```python
from build123d import *

# Parameters (mm, degrees)
SKETCH_1_W               = 27.5
SKETCH_1_H               = 22.5
EXTRUDE_1_DEPTH          = 17.8
CUT_EXTRUDE_1_DEPTH      = 26.148856833
CUT_EXTRUDE_1_DEPTH_BACK = 26.148856833
SKETCH_3_W               = 15.5
SKETCH_3_H               = 12.2
CUT_EXTRUDE_2_DEPTH      = 26.148856833
EXTRUDE_2_DEPTH          = 5.1
EXTRUDE_2_DEPTH_BACK     = 5.1
EXTRUDE_3_DEPTH          = 0.99
EXTRUDE_4_DEPTH          = 0.99
EXTRUDE_5_DEPTH          = 3.01
SKETCH_8_R               = 0.4
EXTRUDE_6_DEPTH          = 2
SKETCH_9_W               = 27.7
SKETCH_9_H               = 18
SKETCH_9_W_2             = 27.5
SKETCH_9_H_2             = 17.8
EXTRUDE_7_DEPTH          = 8.5


with BuildPart() as part:
    # Эскиз1 → Бобышка-Вытянуть1 (new body)
    with BuildSketch(Plane(origin=(0, 0, 0), x_dir=(1, 0, 0), z_dir=(0, 1, 0))):
        Rectangle(SKETCH_1_W, SKETCH_1_H)
    extrude(amount=EXTRUDE_1_DEPTH)

    # Эскиз3 → Вырез-Вытянуть1 (cut, two sides: drawn at the far end of the back side and taken through both)
    with BuildSketch(Plane.XY.offset(-CUT_EXTRUDE_1_DEPTH_BACK)):
        with Locations((0, 8.9)):
            Rectangle(SKETCH_3_W, SKETCH_3_H)
    extrude(amount=CUT_EXTRUDE_1_DEPTH + CUT_EXTRUDE_1_DEPTH_BACK, mode=Mode.SUBTRACT)

    # Эскиз4 → Вырез-Вытянуть2 (cut, through all)
    with BuildSketch(Plane(origin=(0, 0, 0), x_dir=(1, 0, 0), z_dir=(0, 1, 0))):
        Polygon((-4.5, 11.25), (-2.75, 8.75), (2.75, 8.75), (4.5, 11.25), align=None)
        Polygon((4.5, -11.25), (-4.5, -11.25), (-2.75, -8.75), (2.75, -8.75), align=None)
    extrude(amount=CUT_EXTRUDE_2_DEPTH, mode=Mode.SUBTRACT)

    # Эскиз2 → Бобышка-Вытянуть2 (add, two sides: drawn at the far end of the back side and taken through both)
    with BuildSketch(Plane(origin=(0, 8.9, 0), x_dir=(1, 0, 0), z_dir=(0, 1, 0)).offset(-EXTRUDE_2_DEPTH_BACK)):
        with BuildLine():
            Line((-10, -2.5), (-10, 2.5))
            ThreePointArc((-10, 2.5), (0, 12.5), (10, 2.5))
            Line((10, 2.5), (10, -2.5))
            ThreePointArc((10, -2.5), (0, -12.5), (-10, -2.5))
        make_face()
    extrude(amount=EXTRUDE_2_DEPTH + EXTRUDE_2_DEPTH_BACK)

    # Эскиз5 → Бобышка-Вытянуть3 (add)
    with BuildSketch(Plane.XZ.offset(-3.8)):
        with BuildLine():
            Line((7, 11.75), (7, -11.75))
            ThreePointArc((7, -11.75), (6.853553391, -12.103553391), (6.5, -12.25))
            Line((6.5, -12.25), (2.75, -12.25))
            Line((2.75, -12.25), (2.084693312, -9.145235456))
            ThreePointArc((2.084693312, -9.145235456), (1.910130877, -8.861166956), (1.595792105, -8.75))
            Line((1.595792105, -8.75), (-1.595792105, -8.75))
            ThreePointArc((-1.595792105, -8.75), (-1.910130877, -8.861166956), (-2.084693312, -9.145235456))
            Line((-2.084693312, -9.145235456), (-2.75, -12.25))
            Line((-2.75, -12.25), (-6.5, -12.25))
            ThreePointArc((-6.5, -12.25), (-6.853553391, -12.103553391), (-7, -11.75))
            Line((-7, -11.75), (-7, 11.75))
            ThreePointArc((-7, 11.75), (-6.853553391, 12.103553391), (-6.5, 12.25))
            Line((-6.5, 12.25), (-2.75, 12.25))
            Line((-2.75, 12.25), (-2.084693312, 9.145235456))
            ThreePointArc((-2.084693312, 9.145235456), (-1.910130877, 8.861166956), (-1.595792105, 8.75))
            Line((-1.595792105, 8.75), (1.595792105, 8.75))
            ThreePointArc((1.595792105, 8.75), (1.910130877, 8.861166956), (2.084693312, 9.145235456))
            Line((2.084693312, 9.145235456), (2.75, 12.25))
            Line((2.75, 12.25), (6.5, 12.25))
            ThreePointArc((6.5, 12.25), (6.853553391, 12.103553391), (7, 11.75))
        make_face()
    extrude(amount=EXTRUDE_3_DEPTH)

    # Эскиз6 → Бобышка-Вытянуть4 (add)
    with BuildSketch(Plane(origin=(0, 14, 0), x_dir=(1, 0, 0), z_dir=(0, 1, 0))):
        with BuildLine():
            Line((-7, -12.75), (-7, 12.75))
            ThreePointArc((-7, 12.75), (-6.853553391, 13.103553391), (-6.5, 13.25))
            Line((-6.5, 13.25), (-6.2, 13.25))
            ThreePointArc((-6.2, 13.25), (-5.7, 12.75), (-5.2, 13.25))
            Line((-5.2, 13.25), (-3.25, 13.25))
            ThreePointArc((-3.25, 13.25), (-2.896446609, 13.103553391), (-2.75, 12.75))
            Line((-2.75, 12.75), (-2.75, 8.75))
            Line((-2.75, 8.75), (2.75, 8.75))
            Line((2.75, 8.75), (2.75, 12.75))
            ThreePointArc((2.75, 12.75), (2.896446609, 13.103553391), (3.25, 13.25))
            Line((3.25, 13.25), (5.2, 13.25))
            ThreePointArc((5.2, 13.25), (5.7, 12.75), (6.2, 13.25))
            Line((6.2, 13.25), (6.5, 13.25))
            ThreePointArc((6.5, 13.25), (6.853553391, 13.103553391), (7, 12.75))
            Line((7, 12.75), (7, -12.75))
            ThreePointArc((7, -12.75), (6.853553391, -13.103553391), (6.5, -13.25))
            Line((6.5, -13.25), (6.2, -13.25))
            ThreePointArc((6.2, -13.25), (5.7, -12.75), (5.2, -13.25))
            Line((5.2, -13.25), (3.25, -13.25))
            ThreePointArc((3.25, -13.25), (2.896446609, -13.103553391), (2.75, -12.75))
            Line((2.75, -12.75), (2.75, -8.75))
            Line((2.75, -8.75), (-2.75, -8.75))
            Line((-2.75, -8.75), (-2.75, -12.75))
            ThreePointArc((-2.75, -12.75), (-2.896446609, -13.103553391), (-3.25, -13.25))
            Line((-3.25, -13.25), (-5.2, -13.25))
            ThreePointArc((-5.2, -13.25), (-5.7, -12.75), (-6.2, -13.25))
            Line((-6.2, -13.25), (-6.5, -13.25))
            ThreePointArc((-6.5, -13.25), (-6.853553391, -13.103553391), (-7, -12.75))
        make_face()
    extrude(amount=EXTRUDE_4_DEPTH)

    # Эскиз7 → Бобышка-Вытянуть5 (add)
    with BuildSketch(Plane(origin=(0, 14.99, 0), x_dir=(1, 0, 0), z_dir=(0, 1, 0))):
        with BuildLine():
            Line((-7, 11.25), (-2.75, 11.25))
            Line((-2.75, 11.25), (-2.75, 12.75))
            ThreePointArc((-2.75, 12.75), (-2.896446609, 13.103553391), (-3.25, 13.25))
            Line((-3.25, 13.25), (-5.2, 13.25))
            ThreePointArc((-5.2, 13.25), (-5.7, 12.75), (-6.2, 13.25))
            Line((-6.2, 13.25), (-6.5, 13.25))
            ThreePointArc((-6.5, 13.25), (-6.853553391, 13.103553391), (-7, 12.75))
            Line((-7, 12.75), (-7, 11.25))
        make_face()
        with BuildLine():
            Line((7, 11.25), (2.75, 11.25))
            Line((2.75, 11.25), (2.75, 12.75))
            ThreePointArc((2.75, 12.75), (2.896446609, 13.103553391), (3.25, 13.25))
            Line((3.25, 13.25), (5.2, 13.25))
            ThreePointArc((5.2, 13.25), (5.7, 12.75), (6.2, 13.25))
            Line((6.2, 13.25), (6.5, 13.25))
            ThreePointArc((6.5, 13.25), (6.853553391, 13.103553391), (7, 12.75))
            Line((7, 12.75), (7, 11.25))
        make_face()
        with BuildLine():
            Line((7, -11.25), (2.75, -11.25))
            Line((2.75, -11.25), (2.75, -12.75))
            ThreePointArc((2.75, -12.75), (2.896446609, -13.103553391), (3.25, -13.25))
            Line((3.25, -13.25), (5.2, -13.25))
            ThreePointArc((5.2, -13.25), (5.7, -12.75), (6.2, -13.25))
            Line((6.2, -13.25), (6.5, -13.25))
            ThreePointArc((6.5, -13.25), (6.853553391, -13.103553391), (7, -12.75))
            Line((7, -12.75), (7, -11.25))
        make_face()
        with BuildLine():
            Line((-7, -11.25), (-2.75, -11.25))
            Line((-2.75, -11.25), (-2.75, -12.75))
            ThreePointArc((-2.75, -12.75), (-2.896446609, -13.103553391), (-3.25, -13.25))
            Line((-3.25, -13.25), (-5.2, -13.25))
            ThreePointArc((-5.2, -13.25), (-5.7, -12.75), (-6.2, -13.25))
            Line((-6.2, -13.25), (-6.5, -13.25))
            ThreePointArc((-6.5, -13.25), (-6.853553391, -13.103553391), (-7, -12.75))
            Line((-7, -12.75), (-7, -11.25))
        make_face()
    extrude(amount=EXTRUDE_5_DEPTH)

    # Эскиз8 → Бобышка-Вытянуть6 (add)
    with BuildSketch(Plane(origin=(0, 18, 0), x_dir=(1, 0, 0), z_dir=(0, 1, 0))):
        with Locations(Location((4, -12.25, 0), (0, 0, 90))):
            Circle(SKETCH_8_R)
        with Locations(Location((-4, -12.25, 0), (0, 0, 90))):
            Circle(SKETCH_8_R)
        with Locations(Location((-4, 12.25, 0), (0, 0, 90))):
            Circle(SKETCH_8_R)
        with Locations(Location((4, 12.25, 0), (0, 0, 90))):
            Circle(SKETCH_8_R)
    extrude(amount=EXTRUDE_6_DEPTH)

    # Эскиз9 → Бобышка-Вытянуть7 (add, symmetric)
    with BuildSketch(Plane.XY):
        with Locations((0, 8.9)):
            Rectangle(SKETCH_9_W, SKETCH_9_H)
        with Locations((0, 8.9)):
            Rectangle(SKETCH_9_W_2, SKETCH_9_H_2, mode=Mode.SUBTRACT)
    extrude(amount=EXTRUDE_7_DEPTH, both=True)


solid = part.part
```
Geometry: final body of the model. Coordinates: model frame, mm. A direction names the side the tool comes from. Give positions to 0.01 mm unless a question says otherwise; leave off trailing zeros. Write each loop counter-clockwise with the first axis right and the second up, starting at its lowest first coordinate (ties: lowest second). Pieces come first, ordered by that corner, then holes.
1. Pin query (flat end, axial travel): P1, Ø1.4, axis at x = 0, y = 15.5, coming from the -Z side; P2, Ø12, axis at x = -7, z = -4.5, coming from the +Y side; P3, Ø4, axis at x = 4, z = -11.5, coming from the -Y side. Return the tip coordinate at first contact, or that it passes through.
2. Reachability of faces 5 (the flat face through (2.422, 3.312, -10.719)), 6 (the flat face through (-3.64, 1.38, 10.02)), 7 (the flat face through (-5, 3, 12.25)) from +Z, -Z, +X, -X, +Y, -Y: full face, straight path, thin tool, end or side. Return the list, or none.
3. Section query C-C, the plane y = 6.5. Return loops of the section in (x, z).
4. Line query: probe 1 along Z at (x, y) = (3.75, 17.25); probe 2 along Z at (x, y) = (4, 19.25); probe 3 along X at (y, z) = (15.25, 12.25). Output: solid intervals per line, ascending.
5. Section query B-B, the plane z = 6. Return loops of the section in (x, y).
6. Section query A-A, the plane x = -0.25. Return loops of the section in (y, z).
7. Section query D-D, the plane x = -5.7. Count the separate pieces of the cut face and the enclosed holes in it, then the cut area to 3 significant figures.
8. Draft query along X for faces 1 (the flat face through (5, 14, -12)), 2 (the flat face through (10, 9, 11.25)), 3 (the flat face through (-13.85, 9, 0)), 4 (the cylindrical face through (3.88, 18.99, 11.87)). Return one class per face: released by +X, released by -X, zero draft, split by the parting line, or undercut.
Computed:
1. P1: stops at z = -8.75
1. P2: stops at y = 17.9
1. P3: stops at y = 0
2. face 5: -Z, -Y
2. face 6: +Z, -Y
2. face 7: +Z, +X, -X, -Y
3. outline: (-13.85, -8.5) - (-13.75, -8.5) - (-13.75, -11.25) - (-7.75, -11.25) - (-7.75, -8.82) arc R10 ccw to (7.75, -8.82) - (7.75, -11.25) - (13.75, -11.25) - (13.75, -8.5) - (13.85, -8.5) - (13.85, 8.5) - (13.75, 8.5) - (13.75, 11.25) - (7.75, 11.25) - (7.75, 8.82) arc R10 ccw to (-7.75, 8.82) - (-7.75, 11.25) - (-13.75, 11.25) - (-13.75, 8.5) - (-13.85, 8.5) - close
4. probe 1: z = -13.25 to -11.25, -10.18 to 10.18, 11.25 to 13.25
4. probe 2: z = -12.65 to -11.85, 11.85 to 12.65
4. probe 3: x = -7 to -2.75, 2.75 to 7
5. outline: (-13.85, -0.1) - (13.85, -0.1) - (13.85, 17.9) - (-13.85, 17.9) - close; hole (-7.75, 2.8) - (7.75, 2.8) - (7.75, 3.8) - (7, 3.8) - (7, 2.81) - (-7, 2.81) - (-7, 3.8) - (-7.75, 3.8) - close; hole (-7.75, 14) - (-7, 14) - (-7, 14.99) - (7, 14.99) - (7, 14) - (7.75, 14) - (7.75, 15) - (-7.75, 15) - close
6. outline: (-0.1, -8.5) - (0, -8.5) - (0, -8.75) - (2.8, -8.75) - (2.8, 8.75) - (0, 8.75) - (0, 8.5) - (-0.1, 8.5) - close; (2.81, -8.75) - (3.8, -8.75) - (3.8, -12.5) - (14, -12.5) - (14, -8.75) - (14.99, -8.75) - (14.99, 8.75) - (14, 8.75) - (14, 12.5) - (3.8, 12.5) - (3.8, 8.75) - (2.81, 8.75) - close; (15, -8.75) - (17.8, -8.75) - (17.8, -8.5) - (17.9, -8.5) - (17.9, 8.5) - (17.8, 8.5) - (17.8, 8.75) - (15, 8.75) - close
7. separate pieces: 2
7. enclosed holes: 1
7. area: 407 mm2
8. face 1: undercut
8. face 2: zero draft
8. face 3: released by -X
8. face 4: undercut
